Check sheet for the modelled part. Datum: model origin and axes. Units: mm. Coordinates: 2 decimals unless noted, no trailing zeros. Loops run counter-clockwise (first coordinate to the right, second up) from the corner with the lowest first, then second, coordinate; pieces in that order, holes last.
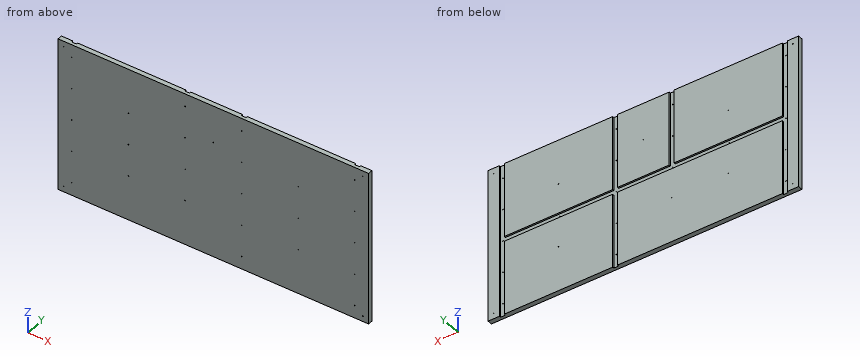
```python
from build123d import *

# Parameters (mm, degrees)
SKETCH1_W               = 1219.2
SKETCH1_H               = 609.6
BOSS_EXTRUDE1_DEPTH     = 18.25625
CUT_EXTRUDE1_DEPTH      = 6.35
SKETCH4_R               = 1.397
CUT_EXTRUDE2_DEPTH      = 7.35
CUT_EXTRUDE2_DEPTH_BACK = 12.90625


with BuildPart() as part:
    # Sketch1 → Boss-Extrude1 (new body)
    with BuildSketch(Plane(origin=(0, 0, 0), x_dir=(1, 0, 0), z_dir=(0, 1, 0))):
        Rectangle(SKETCH1_W, SKETCH1_H)
    extrude(amount=BOSS_EXTRUDE1_DEPTH)

    # Sketch2 → Cut-Extrude1 (cut)
    with BuildSketch(Plane(origin=(0, 18.25625, 0), x_dir=(1, 0, 0), z_dir=(0, 1, 0))):
        Polygon((-565.15, 304.8), (-546.1, 304.8), (-546.1, 9.525), (101.6, 9.525), (101.6, 304.8), (120.65, 304.8), (120.65, 9.525), (546.1, 9.525), (546.1, 304.8), (565.15, 304.8), (565.15, -304.8), (546.1, -304.8), (546.1, -9.525), (120.65, -9.525), (120.65, -304.8), (101.6, -304.8), (101.6, -9.525), (-101.6, -9.525), (-101.6, -304.8), (-120.65, -304.8), (-120.65, -9.525), (-546.1, -9.525), (-546.1, -304.8), (-565.15, -304.8), align=None)
    extrude(amount=-CUT_EXTRUDE1_DEPTH, mode=Mode.SUBTRACT)

    # Sketch4 → Cut-Extrude2 (cut, two sides)
    with BuildSketch(Plane(origin=(0, 11.90625, 0), x_dir=(1, 0, 0), z_dir=(0, 1, 0))) as cut_extrude2_sk:
        with Locations((-555.625, 254)):
            Circle(SKETCH4_R)
        with Locations((111.125, 254)):
            Circle(SKETCH4_R)
        with Locations((555.625, 254)):
            Circle(SKETCH4_R)
        with Locations((-333.375, 127)):
            Circle(SKETCH4_R)
        with Locations((-111.125, 127)):
            Circle(SKETCH4_R)
        with Locations((111.125, 127)):
            Circle(SKETCH4_R)
        with Locations((333.375, 127)):
            Circle(SKETCH4_R)
        with Locations((555.625, 127)):
            Circle(SKETCH4_R)
        with Locations((-333.375, 0)):
            Circle(SKETCH4_R)
        with Locations((-111.125, 0)):
            Circle(SKETCH4_R)
        with Locations((111.125, 0)):
            Circle(SKETCH4_R)
        with Locations((333.375, 0)):
            Circle(SKETCH4_R)
        with Locations((555.625, 0)):
            Circle(SKETCH4_R)
        with Locations((-333.375, -127)):
            Circle(SKETCH4_R)
        with Locations((-111.125, -127)):
            Circle(SKETCH4_R)
        with Locations((111.125, -127)):
            Circle(SKETCH4_R)
        with Locations((333.375, -127)):
            Circle(SKETCH4_R)
        with Locations((555.625, -127)):
            Circle(SKETCH4_R)
        with Locations((-111.125, -254)):
            Circle(SKETCH4_R)
        with Locations((111.125, -254)):
            Circle(SKETCH4_R)
        with Locations((555.625, -254)):
            Circle(SKETCH4_R)
        with Locations((-555.625, 127)):
            Circle(SKETCH4_R)
        with Locations((-555.625, 0)):
            Circle(SKETCH4_R)
        with Locations((-555.625, -127)):
            Circle(SKETCH4_R)
        with Locations((-555.625, -254)):
            Circle(SKETCH4_R)
        with Locations((-587.375, 282.575)):
            Circle(SKETCH4_R)
        with Locations((587.375, 282.575)):
            Circle(SKETCH4_R)
        with Locations((587.375, -282.575)):
            Circle(SKETCH4_R)
        with Locations((-587.375, -282.575)):
            Circle(SKETCH4_R)
        with Locations((0, -157.1625)):
            Circle(SKETCH4_R)
    extrude(amount=CUT_EXTRUDE2_DEPTH, mode=Mode.SUBTRACT)
    extrude(cut_extrude2_sk.sketch, amount=-CUT_EXTRUDE2_DEPTH_BACK, mode=Mode.SUBTRACT)


solid = part.part
```
1) Section check A-A on z = 183. Enter the section's corners in (x, y).
Answer sheet:
outline: (-609.6, 0) - (609.6, 0) - (609.6, 18.26) - (565.15, 18.26) - (565.15, 11.91) - (546.1, 11.91) - (546.1, 18.26) - (120.65, 18.26) - (120.65, 11.91) - (101.6, 11.91) - (101.6, 18.26) - (-101.6, 18.26) - (-101.6, 11.91) - (-120.65, 11.91) - (-120.65, 18.26) - (-546.1, 18.26) - (-546.1, 11.91) - (-565.15, 11.91) - (-565.15, 18.26) - (-609.6, 18.26) - close
2) Scan lines: line 1 (X direction, y = 6.25, z = -254); line 2 (X direction, y = 15.5, z = 195); line 3 (X direction, y = 8.5, z = 254). Record each from-to range of solid material in increasing order.
Answer sheet:
line 1: x = -609.6 to -557.02, -554.23 to 109.73, 112.52 to 554.23, 557.02 to 609.6
line 2: x = -609.6 to -565.15, -546.1 to -120.65, -101.6 to 101.6, 120.65 to 546.1, 565.15 to 609.6
line 3: x = -609.6 to -557.02, -554.23 to -112.52, -109.73 to 109.73, 112.52 to 554.23, 557.02 to 609.6
3) Section check B-B on y = 15.5. Give the number of separate pieces and of enclosed holes in the cut face, plus the area to 3 significant figures.
Answer sheet:
separate pieces: 7
enclosed holes: 10
area: 682,000 mm2
4) Section check C-C on z = -86. Enter the section's corners in (x, y).
Answer sheet:
outline: (-609.6, 0) - (609.6, 0) - (609.6, 18.26) - (565.15, 18.26) - (565.15, 11.91) - (546.1, 11.91) - (546.1, 18.26) - (120.65, 18.26) - (120.65, 11.91) - (101.6, 11.91) - (101.6, 18.26) - (-546.1, 18.26) - (-546.1, 11.91) - (-565.15, 11.91) - (-565.15, 18.26) - (-609.6, 18.26) - close
5) Depth check by flat-ended pin: pin 1 (4.5 mm diameter, centred on x = 111.125, z = 254, fed in from +Y). Enter the tip coordinate at first touch or a pass-through.
Answer sheet:
pin 1: stops at y = 11.91
